Autodesk Inventor part; units mm, degrees
ref_plane "YZ Plane" through (0, 0, 0) normal (1, 0, 0) x (0, 1, 0)
ref_plane "XZ Plane" through (0, 0, 0) normal (0, 1, 0) x (-1, 0, 0)
ref_plane "XY Plane" through (0, 0, 0) normal (0, 0, 1) x (1, 0, 0)
sketch "Sketch1" plane through (0, 0, 0) normal (0, 0, 1) x (1, 0, 0)
  line L0 (-231.775, 155.575) -> (231.775, 155.575)
  line L1 (231.775, 155.575) -> (231.775, -155.575)
  line L2 (231.775, -155.575) -> (-231.775, -155.575)
  line L3 (-231.775, -155.575) -> (-231.775, 155.575)
  line L4 (-231.775, 155.575) -> (231.775, -155.575) construction
  line L5 (231.775, 155.575) -> (-231.775, -155.575) construction
  line L6 (184.15, -107.95) -> (184.15, 107.95)
  line L7 (184.15, 107.95) -> (-184.15, 107.95)
  line L8 (-184.15, 107.95) -> (-184.15, -107.95)
  line L9 (-184.15, -107.95) -> (184.15, -107.95)
  point P0 (0, 0)
  dimension "d0" = 463.55
  dimension "d1" = 311.15
  dimension "d2" = 47.625
extrude "Extrusion1" add sketch "Sketch1" along normal blind 1.397
sketch "Sketch2" plane through (0, 0, 0) normal (0, 0, -1) x (-1, 0, 0)
  line L0 (-231.775, -155.575) -> (-231.775, 155.575)
  line L1 (231.775, -155.575) -> (-231.775, -155.575)
  line L2 (-231.775, -155.575) -> (-231.775, 155.575)
  line L3 (-231.775, 155.575) -> (231.775, 155.575)
  line L4 (231.775, 155.575) -> (231.775, -155.575)
  line L5 (231.775, -155.575) -> (-231.775, 155.575) construction
  line L6 (-231.775, -155.575) -> (231.775, 155.575) construction
  line L7 (230.378, 154.178) -> (-230.378, 154.178)
  line L8 (-230.378, 154.178) -> (-230.378, -154.178)
  line L9 (-230.378, -154.178) -> (230.378, -154.178)
  line L10 (230.378, -154.178) -> (230.378, 154.178)
  point P0 (0, 0)
  dimension "d5" = 1.397
extrude "Extrusion2" add sketch "Sketch2" along normal blind 25.4
properties part number "Top Frame Piece" material "Steel, Mild"
The model under review builds one solid part; all positions refer to its coordinate system, in mm. A direction names the side the tool comes from. Coordinates: 2 decimals unless noted, no trailing zeros. Loops run counter-clockwise (first coordinate to the right, second up) from the corner with the lowest first, then second, coordinate; pieces in that order, holes last. Notation, with made-up numbers: M 67,18.5 L 119,18.5 A25 cw 119,33.5 Z; hole C 22.5,-4 d3. An arc over 180 degrees is marked long. Put each result on its own line as item: value. Start each with the question number.
Q1. Add section C-C (z = -6.25). Write out the cut boundary in (x, y) (3 decimals), and give its area (3 significant figures).
Q2. For faces 5 (the flat face through (230.378, 2, -13)), 6 (the flat face through (-231.775, -2, -12)), list the 3-axis set-ups (+Z, -Z, +X, -X, +Y, -Y) from which the entire face can be reached by the end or side of a thin tool; tool diameter is ignored.
Q3. Add section B-B (y = 44). Write out the cut boundary in (x, z) (3 decimals), and give its area (3 significant figures).
Q4. Add section D-D (x = -196.5). Write out the cut boundary in (y, z) (3 decimals).
Q5. Clearance check with a flat-ended pin moving along its axis: pin 1 (6 mm diameter, centred on x = 85, y = 120.5, fed in from -Z). State where the tip first meets the part, or that it passes through.
Q6. Wall thickness on line 1 (Y direction, x = 186.5, z = -11.5) (3 decimals); line 2 (X direction, y = -53.5, z = -20) (3 decimals); line 3 (Z direction, x = 197.5, y = -11): over which ranges is each line inside the solid? List them lowest first.
Q7. Add section A-A (x = 133). Write out the cut boundary in (y, z) (3 decimals).
Q8. The part is to be moulded in two halves that separate along X. For faces 1 (the flat face through (-3, 154.178, -13)), 2 (the flat face through (3, -154.178, -13)), 3 (the flat face through (231.775, 2, -12)), 4 (the flat face through (-3, 155.575, -12)), say which applies: +X half, -X half, draft (parallel to the pull), parting line (faces both ways), or undercut.
Answers:
1. outline: M -231.775,-155.575 L 231.775,-155.575 L 231.775,155.575 L -231.775,155.575 Z; hole M -230.378,-154.178 L 230.378,-154.178 L 230.378,154.178 L -230.378,154.178 Z
1. area: 2,160 mm^2
2. face 5: -Z
2. face 6: +Z, -Z, -X, +Y, -Y
3. outline: M -231.775,-25.4 L -230.378,-25.4 L -230.378,0 L -184.15,0 L -184.15,1.397 L -231.775,1.397 Z; M 184.15,0 L 230.378,0 L 230.378,-25.4 L 231.775,-25.4 L 231.775,1.397 L 184.15,1.397 Z
3. area: 204 mm^2
4. outline: M -155.575,-25.4 L -154.178,-25.4 L -154.178,0 L 154.178,0 L 154.178,-25.4 L 155.575,-25.4 L 155.575,1.397 L -155.575,1.397 Z
5. pin 1: stops at z = 0
6. line 1: y = -155.575 to -154.178, 154.178 to 155.575
6. line 2: x = -231.775 to -230.378, 230.378 to 231.775
6. line 3: z = 0 to 1.4
7. outline: M -155.575,-25.4 L -154.178,-25.4 L -154.178,0 L -107.95,0 L -107.95,1.397 L -155.575,1.397 Z; M 107.95,0 L 154.178,0 L 154.178,-25.4 L 155.575,-25.4 L 155.575,1.397 L 107.95,1.397 Z
8. face 1: undercut
8. face 2: undercut
8. face 3: +X half
8. face 4: draft
